Source: CAD feature listing. Evaluate the final solid. Frame: model axes, mm. A direction names the side the tool comes from. Give positions to 0.01 mm unless a question says otherwise; leave off trailing zeros. Write each loop counter-clockwise with the first axis right and the second up, starting at its lowest first coordinate (ties: lowest second). Pieces come first, ordered by that corner, then holes. Notation, with made-up numbers: (38, 41.5) -> (97, 41.5) arc R27 ccw to (97, 63.5) -> close; hole circle Ø6 at (71, 39). An arc over 180 degrees is marked (long way). Use one line per item in the form item = value. Start each with the question number.
(1) Cut plane A-A, the plane x = 43. Output: boundary loops of the cut face in (y, z), and give its area (3 significant figures).
(2) Cut plane B-B, the plane x = 29.5. Output: boundary loops of the cut face in (y, z).
(3) Draft query along Y for faces 1 (the face through (46.3, 2, 0)), 2 (the face through (51.6, -2, -2)), 3 (the face through (7.52, -1.5, 0.07)). Return one class per face: pulls with the +Y half, pulls with the -Y half, needs draft (parallel to the pull), parting line crosses it, or undercut.
(4) Set-up query: faces 4 (the face through (50.42, -1.93, -8.69)), 5 (the face through (3.3, 4, -2)), 6 (the face through (0, -2, 2)), 7 (the face through (52.586, 1.846, -3.549)), 8 (the face through (53.6, -4, 2)). Return all of +Z, -Z, +X, -X, +Y, -Y with unobstructed straight access to the full face (end or side cutting, diameter ignored); none if empty.
(5) Material intervals for line 1 along X through (y, z) = (-1.5, -3); line 2 along X through (y, z) = (-4, 1.5); line 3 along Y through (x, z) = (-0.9, 0), sorted ascending. Write a range as from..to.
(6) First-contact query: P1, Ø0.6, axis at x = 51.5, z = -1.5, coming from the -Y side; P2, Ø0.6, axis at x = 52, y = -2.5, coming from the -Z side; P3, Ø2.5, axis at y = 1.5, z = -2.5, coming from the -X side; P4, Ø2, axis at x = 17, z = 2.5, coming from the +Y side. Flat tips, straight axial feed; report the tip coordinate or a pass-through.
from build123d import *

# Parameters (mm, degrees)
SKETCH_R      = 8.9
PAD_DEPTH     = 3.3
SKETCH001_R   = 8.9
SKETCH001_R_2 = 4
PAD001_DEPTH  = 2
SKETCH003_R   = 4
PAD002_DEPTH  = 2
SKETCH004_R   = 1.5
PAD003_DEPTH  = 4.5
SKETCH005_R   = 1.9
PAD004_DEPTH  = 32
FILLET_R      = 1
SKETCH006_R   = 1.5
PAD005_DEPTH  = 4.5
SKETCH007_R   = 4
PAD006_DEPTH  = 2
SKETCH008_R   = 8.9
PAD007_DEPTH  = 3.3
SKETCH009_R   = 8.9
SKETCH009_R_2 = 4
PAD008_DEPTH  = 2
FILLET001_R   = 1
FILLET002_R   = 0.2
FILLET003_R   = 0.2
PAD009_DEPTH  = 0.5
PAD010_DEPTH  = 0.5


with BuildPart() as part:
    # Sketch → Pad (new body)
    with BuildSketch(Plane.YZ):
        Circle(SKETCH_R)
    extrude(amount=PAD_DEPTH)

    # Sketch001 (on Face2 of Pad) → Pad001 (join)
    with BuildSketch(Plane(origin=(0, 0, 0), x_dir=(0, 1, 0), z_dir=(-1, 0, 0))):
        Circle(SKETCH001_R)
        Circle(SKETCH001_R_2, mode=Mode.SUBTRACT)
    extrude(amount=PAD001_DEPTH)

    # Sketch003 (on Face3 of Pad001) → Pad002 (join)
    with BuildSketch(Plane.YZ.offset(3.3)):
        Circle(SKETCH003_R)
    extrude(amount=PAD002_DEPTH)

    # Sketch004 (on Face7 of Pad002) → Pad003 (join)
    with BuildSketch(Plane.YZ.offset(5.3)):
        Circle(SKETCH004_R)
    extrude(amount=PAD003_DEPTH)

    # Sketch005 (on Face10 of Pad003) → Pad004 (join)
    with BuildSketch(Plane.YZ.offset(9.8)):
        Circle(SKETCH005_R)
    extrude(amount=PAD004_DEPTH)

    # Fillet
    fillet_edges = [part.edges().sort_by_distance(p)[0] for p in [
        (-2, -8.9, 0),
    ]]
    fillet(fillet_edges, radius=FILLET_R)

    # Sketch006 (on Face13 of Fillet) → Pad005 (join)
    with BuildSketch(Plane.YZ.offset(41.8)):
        Circle(SKETCH006_R)
    extrude(amount=PAD005_DEPTH)

    # Sketch007 (on Face15 of Pad005) → Pad006 (join)
    with BuildSketch(Plane.YZ.offset(46.3)):
        Circle(SKETCH007_R)
    extrude(amount=PAD006_DEPTH)

    # Sketch008 (on Face3 of Pad006) → Pad007 (join)
    with BuildSketch(Plane.YZ.offset(48.3)):
        Circle(SKETCH008_R)
    extrude(amount=PAD007_DEPTH)

    # Sketch009 (on Face3 of Pad007) → Pad008 (join)
    with BuildSketch(Plane.YZ.offset(51.6)):
        Circle(SKETCH009_R)
        Circle(SKETCH009_R_2, mode=Mode.SUBTRACT)
    extrude(amount=PAD008_DEPTH)

    # Fillet001
    fillet001_edges = [part.edges().sort_by_distance(p)[0] for p in [
        (53.6, -8.9, 0),
    ]]
    fillet(fillet001_edges, radius=FILLET001_R)

    # Fillet002
    fillet002_edges = [part.edges().sort_by_distance(p)[0] for p in [
        (41.8, -1.9, 0),
    ]]
    fillet(fillet002_edges, radius=FILLET002_R)

    # Fillet003
    fillet003_edges = [part.edges().sort_by_distance(p)[0] for p in [
        (9.8, -1.9, 0),
    ]]
    fillet(fillet003_edges, radius=FILLET003_R)

    # Sketch010 (on Face24 of Fillet003) → Pad009 (join)
    with BuildSketch(Plane(origin=(0, 0, 0), x_dir=(0, 1, 0), z_dir=(-1, 0, 0))):
        Polygon((-0.6, 0.6), (-0.6, 4), (0.6, 4), (0.6, 0.6), (4, 0.6), (4, -0.6), (0.6, -0.6), (0.6, -4), (-0.6, -4), (-0.6, -0.6), (-4, -0.6), (-4, 0.6), align=None)
    extrude(amount=PAD009_DEPTH)

    # Sketch011 (on Face37 of Pad009) → Pad010 (join)
    with BuildSketch(Plane.YZ.offset(51.6)):
        Polygon((-0.6, -0.6), (-0.6, -4), (0.6, -4), (0.6, -0.6), (4, -0.6), (4, 0.6), (0.6, 0.6), (0.6, 4), (-0.6, 4), (-0.6, 0.6), (-4, 0.6), (-4, -0.6), align=None)
    extrude(amount=PAD010_DEPTH)


solid = part.part
Geometry says:
q1.outline = circle Ø3 at (0, 0)
q1.area = 7.07 mm^2
q2.outline = circle Ø3.8 at (0, 0)
q3.face_1 = needs draft
q3.face_2 = undercut
q3.face_3 = parting line crosses it
q4.face_4 = +X, -X
q4.face_5 = none
q4.face_6 = -X
q4.face_7 = +X
q4.face_8 = +Z, -Z, +X, +Y, -Y
q5.line_1 = 0..5.3, 46.3..51.6
q5.line_2 = -2..3.3, 48.3..53.6
q5.line_3 = -8.9..-4, 4..8.9
q6.P1 = -8.82
q6.P2 = -8.62
q6.P3 = -2
q6.P4 = 1.17
